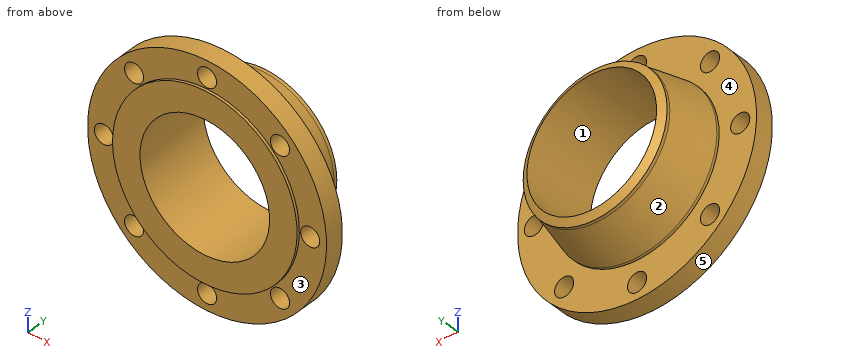
```python
from build123d import *

# Parameters (mm, degrees)
F2_R     = 11.19886
F3_DEPTH = 85.726


with BuildPart() as f1:
    # F0 (on Right) → F1 (revolve)
    with BuildSketch(Plane.YZ):
        Polygon((0, 107.95), (0, 75.82916), (88.9, 75.82916), (84.116041, 84.19973), (80.306041, 84.19973), (28.575, 95.9993), (25.4, 95.9993), (25.4, 139.74953), (3.175, 139.74953), (3.175, 107.95), align=None)
    revolve(axis=Axis((0, -0.252383, 0), (0, 1, 0)))

    # F2 (on face) → F3 (cut, through all)
    with BuildSketch(Plane.XZ.offset(-3.175)):
        with Locations((-85.312433, 85.312433)):
            Circle(F2_R)
        with Locations((0, 120.65)):
            Circle(F2_R)
        with Locations((85.312433, 85.312433)):
            Circle(F2_R)
        with Locations((120.65, 0)):
            Circle(F2_R)
        with Locations((85.312433, -85.312433)):
            Circle(F2_R)
        with Locations((0, -120.65)):
            Circle(F2_R)
        with Locations((-85.312433, -85.312433)):
            Circle(F2_R)
        with Locations((-120.65, 0)):
            Circle(F2_R)
    extrude(amount=-F3_DEPTH, mode=Mode.SUBTRACT)


solid = f1.part
```
Here's how the part is built. I have some questions about the finished solid (model axes, mm). Face numbers are marked on the shaded views. A direction names the side the tool comes from. Coordinates: 2 decimals unless noted, no trailing zeros. Order: outer loops, then holes, each group sorted by start corner. A loop starts at its lowest first (then second) coordinate and runs counter-clockwise, first axis right, second up.
1) I need wall thicknesses on line 1 (Y direction, x = 54, z = -107.5) (3 decimals); line 2 (Z direction, x = 4.5, y = 23.5); line 3 (X direction, y = 13, z = 50.5). Which ranges of each line are inside material? Lowest first, please.
2) Imagine slicing it at C-C on x = -114.5. List the corners of the cut face in (y, z) for me (3 decimals).
3) Imagine slicing it at A-A on x = 0. List the corners of the cut face in (y, z) for me (3 decimals).
4) We'd pull the mould along Z, two halves only. Please class the marked faces 1, 2 and 3: +Z half, -Z half, draft (parallel to the pull), parting line (faces both ways), or undercut.
5) Imagine slicing it at D-D on z = 120.65. List the corners of the cut face in (x, y) for me (3 decimals), and give its area (3 significant figures).
6) Which directions (+Z, -Z, +X, -X, +Y, -Y) give clear straight access to the entire face, cutting with the end or side of a thin tool? Please do the marked faces 4 and 5.
7) Imagine slicing it at B-B on z = 0. List the corners of the cut face in (x, y) for me (3 decimals).
8) Will these pins go through, and if not, where does the flat tip stop? pin 1 (1.5 mm diameter, centred on x = -26.5, z = -74.5, fed in from +Y); pin 2 (4 mm diameter, centred on x = 68, z = -41.5, fed in from -Y); pin 3 (8 mm diameter, centred on y = 16, z = 57.5, fed in from -X); pin 4 (10 mm diameter, centred on y = 59.5, z = 43, fed in from +X).
Response values:
1. line 1: y = 3.175 to 25.4
1. line 2: z = -139.68 to -130.9, -110.4 to -75.7, 75.7 to 110.4, 130.9 to 139.68
1. line 3: x = -130.31 to -56.57, 56.57 to 130.31
2. outline: (3.175, -80.123) - (25.4, -80.123) - (25.4, -9.359) - (3.175, -9.359) - close; (3.175, 9.359) - (25.4, 9.359) - (25.4, 80.123) - (3.175, 80.123) - close
3. outline: (0, -107.95) - (3.175, -107.95) - (3.175, -109.451) - (25.4, -109.451) - (25.4, -95.999) - (28.575, -95.999) - (80.306, -84.2) - (84.116, -84.2) - (88.9, -75.829) - (0, -75.829) - close; (0, 75.829) - (88.9, 75.829) - (84.116, 84.2) - (80.306, 84.2) - (28.575, 95.999) - (25.4, 95.999) - (25.4, 109.451) - (3.175, 109.451) - (3.175, 107.95) - (0, 107.95) - close; (3.175, -139.75) - (25.4, -139.75) - (25.4, -131.849) - (3.175, -131.849) - close; (3.175, 131.849) - (25.4, 131.849) - (25.4, 139.75) - (3.175, 139.75) - close
4. face 1: undercut
4. face 2: parting line
4. face 3: draft
5. outline: (-70.523, 3.175) - (-11.199, 3.175) - (-11.199, 25.4) - (-70.523, 25.4) - close; (11.199, 3.175) - (70.523, 3.175) - (70.523, 25.4) - (11.199, 25.4) - close
5. area: 2,640 mm2
6. face 4: +Y
6. face 5: +Y, -Y
7. outline: (-139.75, 3.175) - (-131.849, 3.175) - (-131.849, 25.4) - (-139.75, 25.4) - close; (-109.451, 3.175) - (-107.95, 3.175) - (-107.95, 0) - (-75.829, 0) - (-75.829, 88.9) - (-84.2, 84.116) - (-84.2, 80.306) - (-95.999, 28.575) - (-95.999, 25.4) - (-109.451, 25.4) - close; (75.829, 0) - (107.95, 0) - (107.95, 3.175) - (109.451, 3.175) - (109.451, 25.4) - (95.999, 25.4) - (95.999, 28.575) - (84.2, 80.306) - (84.2, 84.116) - (75.829, 88.9) - close; (131.849, 3.175) - (139.75, 3.175) - (139.75, 25.4) - (131.849, 25.4) - close
8. pin 1: stops at y = 87.47
8. pin 2: stops at y = 0
8. pin 3: stops at x = -129.1
8. pin 4: stops at x = 80.73
